Source: three-view drawing plus pictorial views. Frame: mm from the lowest corner of the part. Round coordinates to 2 decimals unless told otherwise and drop trailing zeros. Write each loop counter-clockwise with the first axis right and the second up, starting at its lowest first coordinate (ties: lowest second). Pieces come first, ordered by that corner, then holes. Notation, with made-up numbers: M 35.25,-9.75 L 50.25,-9.75 A21 ccw 50.25,11.25 Z; hole C 44,-26.75 d9. An arc over 180 degrees is marked long. Answer as CSV lines item,"result". Start each with the question number.
Q1. Ray query, probe 1 along Z at (x, y) = (19, 18.5). Return the intervals inside material, ascending.
Q2. Section query C-C on x = 39.5. Output: boundary loops of the cut face in (y, z), and give its area (3 significant figures).
Q3. Section query A-A on x = 30.5. Output: boundary loops of the cut face in (y, z), and give its area (4 significant figures).
Q4. First-contact query: pin 1 (4 mm diameter, centred on y = 61.5, z = 58.5, fed in from -X); pin 2 (1.5 mm diameter, centred on x = 41, y = 33, fed in from +Z); pin 3 (1.5 mm diameter, centred on x = 25.5, z = 57.5, fed in from -Y). Flat tips, straight axial feed; report the tip coordinate or a pass-through.
Q5. Section query B-B on y = 28.5. Output: boundary loops of the cut face in (x, z), and give its area (4 significant figures).
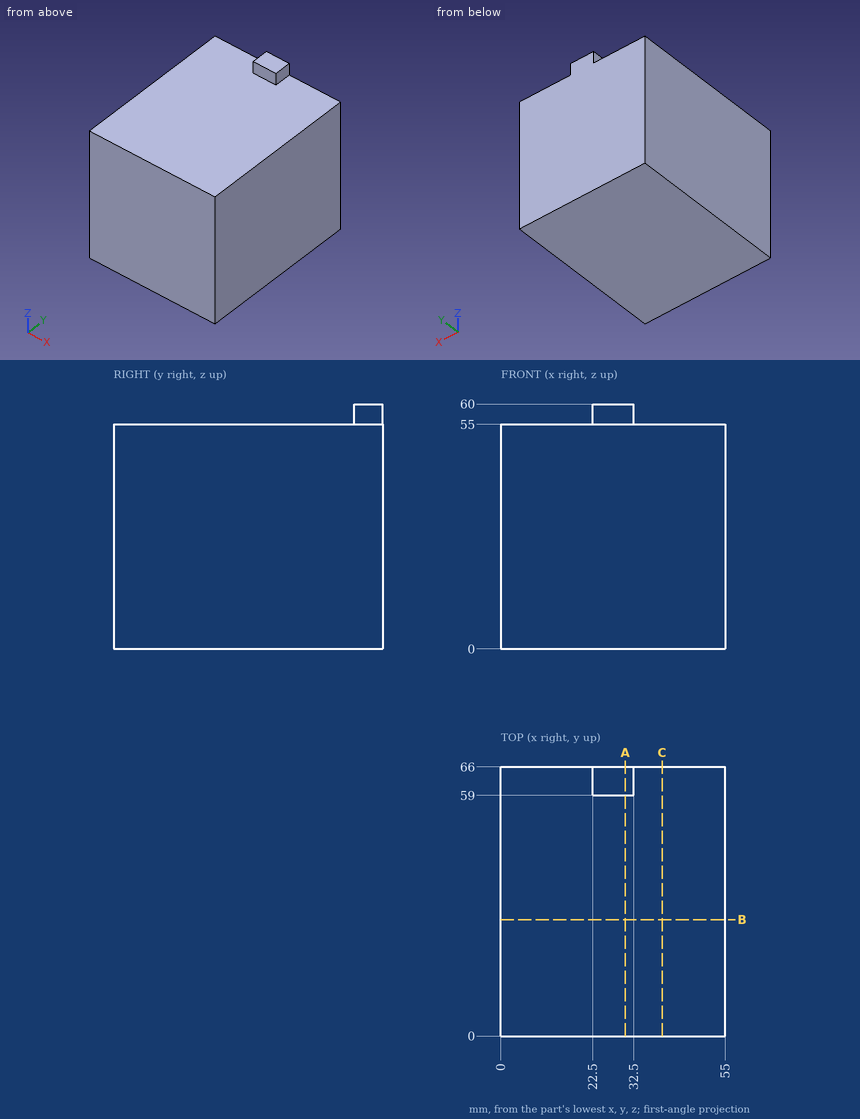
Entries:
1,probe 1,"z = 0 to 55"
2,outline,"M 0,0 L 66,0 L 66,55 L 0,55 Z"
2,area,"3,630 mm^2"
3,outline,"M 0,0 L 66,0 L 66,60 L 59,60 L 59,55 L 0,55 Z"
3,area,"3,665 mm^2"
4,pin 1,"stops at x = 22.5"
4,pin 2,"stops at z = 55"
4,pin 3,"stops at y = 59"
5,outline,"M 0,0 L 55,0 L 55,55 L 0,55 Z"
5,area,"3,025 mm^2"
